from build123d import *

# Parameters (mm, degrees)
F0_W          = 12.7
F0_H          = 3.175
F0_H_2        = 12.7
F1_DEPTH      = 27.94
F2_W          = 12.7
F2_H          = 10.9347
F2_H_2        = 3.0353
F3_DEPTH      = 7.62
F4_W          = 12.7
F4_H          = 13.97
F5_DEPTH      = 7.62
F7_DEPTH      = 25.4
F10_DEPTH     = 25.4
F11_T1_DEPTH  = 44.45
F12_R         = 6.35
F13_R         = 6.35
F14_T1_DEPTH  = 15.24
F14_T3_DEPTH  = 1.905
F14_T6_ANGLE  = 90
F14_T8_ANGLE  = 90
F14_T10_ANGLE = 90
F14_T12_ANGLE = 90


# Not quite as in the source:
# - a fillet or chamfer that OpenCascade refuses, or shapes differently, is made with other operations: its cross-section is extruded or revolved along the edge and cut away or added


with BuildPart() as f1:
    # F0 (on Front) → F1 (new body)
    with BuildSketch(Plane.XZ):
        with Locations((-19.05, 11.1125)):
            Rectangle(F0_W, F0_H)
        with Locations((-19.05, 19.05)):
            Rectangle(F0_W, F0_H_2)
    extrude(amount=F1_DEPTH)

    # F2 (on face) → F3 (join)
    with BuildSketch(Plane.XY.offset(25.4)):
        with Locations((-19.05, -33.40735)):
            Rectangle(F2_W, F2_H)
        with Locations((-19.05, -40.39235)):
            Rectangle(F2_W, F2_H_2)
    extrude(amount=-F3_DEPTH)

    # F4 (on face) → F5 (join)
    with BuildSketch(Plane.XY.offset(25.4)):
        with Locations((-19.05, 6.985)):
            Rectangle(F4_W, F4_H)
    extrude(amount=-F5_DEPTH)

    # F6 (on face) → F7 (cut)
    with BuildSketch(Plane(origin=(-25.4, 0, 0), x_dir=(0, -1, 0), z_dir=(-1, 0, 0))):
        with BuildLine():
            ThreePointArc((1.27, 25.4), (13.97, 12.7), (26.67, 25.4))
            Line((26.67, 25.4), (1.27, 25.4))
        make_face()
    extrude(amount=-F7_DEPTH, mode=Mode.SUBTRACT)

    # F8 (on face) + F9 (on face) → F10 (cut)
    with BuildSketch(Plane(origin=(0, 0, 17.78), x_dir=(1, 0, 0), z_dir=(0, 0, -1))):
        with BuildLine():
            ThreePointArc((-19.05, 38.735), (-21.2950640303, 33.3149359697), (-15.875, 35.56))
            ThreePointArc((-15.875, 35.56), (-16.8049359697, 37.8050640303), (-19.05, 38.735))
        make_face()
    with BuildSketch(Plane(origin=(0, 0, 17.78), x_dir=(1, 0, 0), z_dir=(0, 0, -1))):
        with BuildLine():
            ThreePointArc((-19.05, -10.795), (-16.8049359697, -9.8650640303), (-15.875, -7.62))
            ThreePointArc((-15.875, -7.62), (-21.2950640303, -5.3749359697), (-19.05, -10.795))
        make_face()
    extrude(amount=-F10_DEPTH, mode=Mode.SUBTRACT)

    # F11: fillet of radius 6.35 on 2 edges, made by hand

    # F11_s2 → F11_t1 (cut)
    with BuildSketch(Plane.YZ.offset(-41.275)):
        with BuildLine():
            ThreePointArc((-35.56, 17.78), (-40.0501280605, 19.6398719395), (-41.91, 24.13))
            Line((-41.91, 24.13), (-41.91, 17.78))
            Line((-41.91, 17.78), (-35.56, 17.78))
        make_face()
        with BuildLine():
            ThreePointArc((13.97, 24.13), (12.1101280605, 19.6398719395), (7.62, 17.78))
            Line((7.62, 17.78), (13.97, 17.78))
            Line((13.97, 17.78), (13.97, 24.13))
        make_face()
    extrude(amount=F11_T1_DEPTH, mode=Mode.SUBTRACT)

    # F12
    f12_edges = [f1.edges().sort_by_distance(p)[0] for p in [
        (-19.05, 0, 9.525),
    ]]
    fillet(f12_edges, radius=F12_R)

    # F13
    f13_edges = [f1.edges().sort_by_distance(p)[0] for p in [
        (-19.05, -27.94, 9.525),
    ]]
    fillet(f13_edges, radius=F13_R)

    # F14: fillet of radius 5.08 on 2 edges, made by hand

    # F14_s2 → F14_t1 (cut)
    with BuildSketch(Plane.XZ.offset(6.35)):
        with BuildLine():
            ThreePointArc((-17.78, 9.525), (-14.1878975516, 11.0128975516), (-12.7, 14.605))
            Line((-12.7, 14.605), (-12.7, 9.525))
            Line((-12.7, 9.525), (-17.78, 9.525))
        make_face()
        with BuildLine():
            ThreePointArc((-20.32, 9.525), (-23.9121024484, 11.0128975516), (-25.4, 14.605))
            Line((-25.4, 14.605), (-25.4, 9.525))
            Line((-25.4, 9.525), (-20.32, 9.525))
        make_face()
    extrude(amount=F14_T1_DEPTH, mode=Mode.SUBTRACT)

    # F14_s4 → F14_t3 (cut)
    with BuildSketch(Plane.XY.offset(15.875)):
        with BuildLine():
            ThreePointArc((-25.4, -22.86), (-23.9121024484, -26.4521024484), (-20.32, -27.94))
            Line((-20.32, -27.94), (-25.4, -27.94))
            Line((-25.4, -27.94), (-25.4, -22.86))
        make_face()
        with BuildLine():
            ThreePointArc((-25.4, -5.08), (-23.9121024484, -1.4878975516), (-20.32, 0))
            Line((-20.32, 0), (-25.4, 0))
            Line((-25.4, 0), (-25.4, -5.08))
        make_face()
        with BuildLine():
            ThreePointArc((-12.7, -22.86), (-14.1878975516, -26.4521024484), (-17.78, -27.94))
            Line((-17.78, -27.94), (-12.7, -27.94))
            Line((-12.7, -27.94), (-12.7, -22.86))
        make_face()
        with BuildLine():
            ThreePointArc((-12.7, -5.08), (-14.1878975516, -1.4878975516), (-17.78, 0))
            Line((-17.78, 0), (-12.7, 0))
            Line((-12.7, 0), (-12.7, -5.08))
        make_face()
    extrude(amount=F14_T3_DEPTH, mode=Mode.SUBTRACT)

    # F14_s5 → F14_t6 (revolve, cut)
    with BuildSketch(Plane.XZ.offset(6.35)):
        with BuildLine():
            ThreePointArc((-25.4, 14.605), (-23.9121024484, 11.0128975516), (-20.32, 9.525))
            Line((-20.32, 9.525), (-25.4, 9.525))
            Line((-25.4, 9.525), (-25.4, 14.605))
        make_face()
    revolve(axis=Axis((-25.4, -6.35, 15.875), (1, 0, 0)), revolution_arc=F14_T6_ANGLE, mode=Mode.SUBTRACT)

    # F14_s7 → F14_t8 (revolve, cut)
    with BuildSketch(Plane.XZ.offset(21.59)):
        with BuildLine():
            ThreePointArc((-25.4, 14.605), (-23.9121024484, 11.0128975516), (-20.32, 9.525))
            Line((-20.32, 9.525), (-25.4, 9.525))
            Line((-25.4, 9.525), (-25.4, 14.605))
        make_face()
    revolve(axis=Axis((-25.4, -21.59, 15.875), (-1, 0, 0)), revolution_arc=F14_T8_ANGLE, mode=Mode.SUBTRACT)

    # F14_s9 → F14_t10 (revolve, cut)
    with BuildSketch(Plane.XZ.offset(6.35)):
        with BuildLine():
            ThreePointArc((-17.78, 9.525), (-14.1878975516, 11.0128975516), (-12.7, 14.605))
            Line((-12.7, 14.605), (-12.7, 9.525))
            Line((-12.7, 9.525), (-17.78, 9.525))
        make_face()
    revolve(axis=Axis((-12.7, -6.35, 15.875), (1, 0, 0)), revolution_arc=F14_T10_ANGLE, mode=Mode.SUBTRACT)

    # F14_s11 → F14_t12 (revolve, cut)
    with BuildSketch(Plane.XZ.offset(21.59)):
        with BuildLine():
            ThreePointArc((-17.78, 9.525), (-14.1878975516, 11.0128975516), (-12.7, 14.605))
            Line((-12.7, 14.605), (-12.7, 9.525))
            Line((-12.7, 9.525), (-17.78, 9.525))
        make_face()
    revolve(axis=Axis((-12.7, -21.59, 15.875), (-1, 0, 0)), revolution_arc=F14_T12_ANGLE, mode=Mode.SUBTRACT)


solid = f1.part
Build history of the part. All positions in model axes, mm. A direction names the side the tool comes from. Coordinates: 2 decimals unless noted, no trailing zeros. Order: outer loops, then holes, each group sorted by start corner. A loop starts at its lowest first (then second) coordinate and runs counter-clockwise, first axis right, second up. Notation, with made-up numbers: (75, 61.5) -> (112, 61.5) arc R17 cw to (112, 72.5) -> close; hole circle Ø1 at (16.5, 46). An arc over 180 degrees is marked (long way). One line per item, written item: value.
(1) Probe line 1 (X direction, y = 7.62, z = 20) (3 decimals); line 2 (Y direction, x = -19.05, z = 21.75) (3 decimals); line 3 (Y direction, x = -19.05, z = 22.25) (3 decimals). List the from-to ranges inside material, lowest first. Write a range as [from, to].
Checked values:
line 1: [-25.4, -22.225], [-15.875, -12.7]
line 2: [-41.447, -38.735], [-32.385, -26.134], [-1.806, 4.445], [10.795, 13.507]
line 3: [-41.625, -38.735], [-32.385, -26.273], [-1.667, 4.445], [10.795, 13.685]
(2) Slice it at B-B, the plane y = -13.97. List the corners of the cut face in (x, z) (3 decimals), plus the area to 3 significant figures.
Checked values:
outline: (-25.029, 12.7) arc R5.08 ccw to (-20.32, 9.525) -> (-17.78, 9.525) arc R5.08 ccw to (-13.071, 12.7) -> close
area: 29.7 mm2
(3) Slice it at A-A, the plane z = 22. List the corners of the cut face in (x, y) (3 decimals), plus the area to 3 significant figures.
Checked values:
outline: (-25.4, -41.542) -> (-12.7, -41.542) -> (-12.7, -26.206) -> (-25.4, -26.206) -> close; (-25.4, -1.734) -> (-12.7, -1.734) -> (-12.7, 13.602) -> (-25.4, 13.602) -> close; hole circle Ø6.35 at (-19.05, -35.56); hole circle Ø6.35 at (-19.05, 7.62)
area: 326 mm2
(4) Drop flat-ended pins along their axis: pin 1 Ø1 at (y, z) = (-8, 13.5) entering from +X; pin 2 Ø2 at (x, z) = (-19.5, 16.5) entering from -Y; pin 3 Ø1.5 at (x, z) = (-19.5, 16.5) entering from +Y. Give the stop position or say it passes through.
Checked values:
pin 1: x = -12.74
pin 2: y = -27.94
pin 3: y = 0
(5) Tool access for faces 1 (the flat face through (-25.4, -22, 15)), 2 (the cylindrical face through (-23.951, -1.528, 16.814)), 3 (the cylindrical face through (-14.149, -26.412, 16.814)), 4 (the flat face through (-19, -27.94, 17)), 5 (the flat face through (-19, 0, 17)): list every direction of +Z, -Z, +X, -X, +Y, -Y with a clear straight run to the whole face (end or side of a thin tool).
Checked values:
face 1: +Z, -Z, -X, +Y, -Y
face 2: -Z, -X, +Y
face 3: -Z, +X, -Y
face 4: -Z, +X, -X, -Y
face 5: -Z, +X, -X, +Y
